Geometry check sheet. Reference: drawing and pictorial views, mm from the part's lowest x, y, z. A direction names the side the tool comes from. Give positions to 0.01 mm unless a question says otherwise; leave off trailing zeros. Order: outer loops, then holes, each group sorted by start corner. A loop starts at its lowest first (then second) coordinate and runs counter-clockwise, first axis right, second up. Notation, with made-up numbers: (78, 79.5) -> (102, 79.5) arc R18 cw to (102, 105.5) -> close; hole circle Ø3 at (-22.5, 38.5). An arc over 180 degrees is marked (long way). Write each question's results on one line, items separated by ' | '.
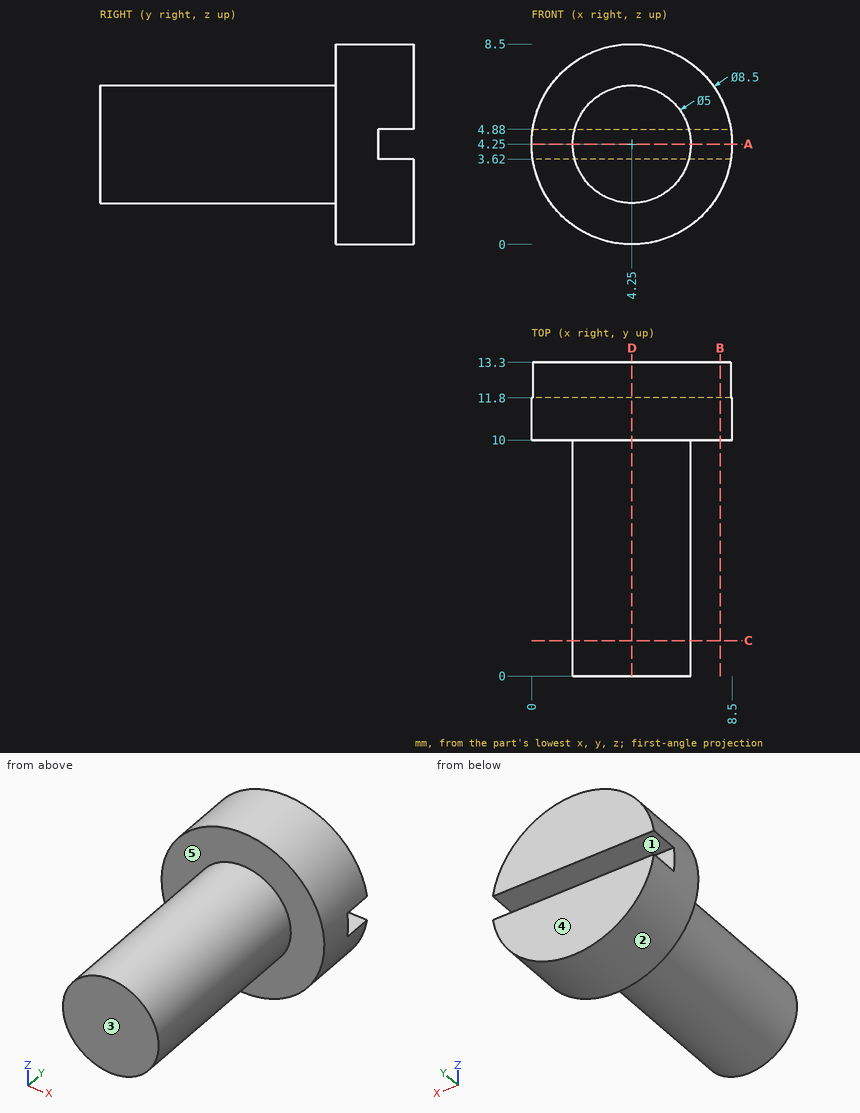
1. Gauge pin test, flat ends, axial feed: pin 1 Ø5 at (y, z) = (8.5, 7) entering from +X; pin 2 Ø1 at (x, y) = (7, 3) entering from +Z; pin 3 Ø5 at (y, z) = (11, 7) entering from -X. Record the tip position at first contact, or that the pin passes through.
Verdict:
pin 1: stops at x = 8.43 | pin 2: stops at z = 5.34 | pin 3: stops at x = 0.01
2. Section check A-A on z = 4.25. Record the cut outline in (x, y).
Verdict:
outline: (0, 10) -> (1.75, 10) -> (1.75, 0) -> (6.75, 0) -> (6.75, 10) -> (8.5, 10) -> (8.5, 11.8) -> (0, 11.8) -> close
3. Section check D-D on x = 4.25. Record the cut outline in (y, z), then the cut area to 3 significant figures.
Verdict:
outline: (0, 1.75) -> (10, 1.75) -> (10, 0) -> (13.3, 0) -> (13.3, 3.62) -> (11.8, 3.62) -> (11.8, 4.88) -> (13.3, 4.88) -> (13.3, 8.5) -> (10, 8.5) -> (10, 6.75) -> (0, 6.75) -> close | area: 76.2 mm^2
4. Mould release check, pull along Z, two halves, no side actions. Record for the marked faces 1, 2 and 3: +Z half, -Z half, draft (parallel to the pull), parting line (faces both ways), or undercut.
Verdict:
face 1: undercut | face 2: parting line | face 3: draft
5. Material ranges on probe 1 along Y at (x, z) = (1.25, 3); probe 2 along Y at (x, z) = (6, 4); probe 3 along Z at (x, y) = (1.5, 13), recorded low to high. Write a range as from..to.
Verdict:
probe 1: y = 10..13.3 | probe 2: y = 0..11.8 | probe 3: z = 1.01..3.62, 4.88..7.49
6. Access from +Z, -Z, +X, -X, +Y, -Y to the whole of each face (thin tool, end or side, straight path). Record for the marked faces 4 and 5.
Verdict:
face 4: +Z, -Z, +X, -X, +Y | face 5: -Y
7. Section check C-C on y = 1.5. Record the cut outline in (x, z).
Verdict:
outline: circle Ø5 at (4.25, 4.25)
8. Section check B-B on x = 8. Record the cut outline in (y, z).
Verdict:
outline: (10, 2.25) -> (13.3, 2.25) -> (13.3, 3.62) -> (11.8, 3.62) -> (11.8, 4.88) -> (13.3, 4.88) -> (13.3, 6.25) -> (10, 6.25) -> close
